Here's how the part is built. I have some questions about the finished solid (model axes, mm). Give positions to 0.01 mm unless a question says otherwise; leave off trailing zeros. Write each loop counter-clockwise with the first axis right and the second up, starting at its lowest first coordinate (ties: lowest second). Pieces come first, ordered by that corner, then holes. Notation, with made-up numbers: (10.5, -8.75) -> (19.5, -8.75) arc R15 cw to (19.5, 1.25) -> close; hole circle Ø11 at (44, -8.75). An arc over 180 degrees is marked (long way). Return JSON: item names as keys, results as strings.
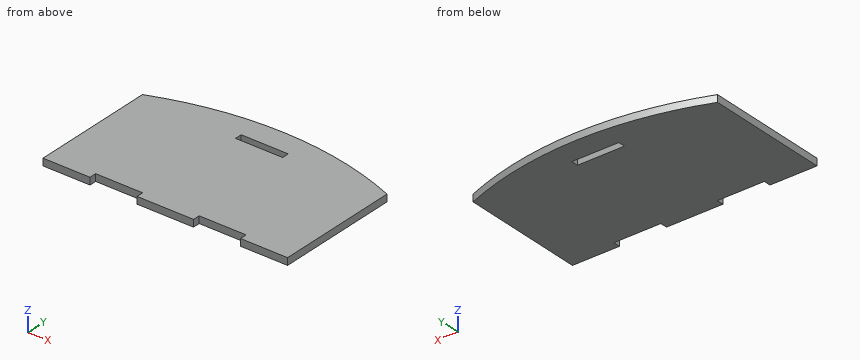
from build123d import *

# Parameters (mm, degrees)
SKETCH1_W           = 20
SKETCH1_H           = 3
BOSS_EXTRUDE1_DEPTH = 3


with BuildPart() as part:
    # Sketch1 → Boss-Extrude1 (new body)
    with BuildSketch(Plane.XY):
        with BuildLine():
            Line((-9.242159986, -25.403689193), (-9.242159986, -22.403689193))
            Line((-9.242159986, -22.403689193), (10.757840014, -22.403689193))
            Line((10.757840014, -22.403689193), (10.757840014, -25.403689193))
            Line((10.757840014, -25.403689193), (34.757840014, -25.403689193))
            Line((34.757840014, -25.403689193), (34.757840014, -22.403689193))
            Line((34.757840014, -22.403689193), (54.757840014, -22.403689193))
            Line((54.757840014, -22.403689193), (54.757840014, -25.403689193))
            Line((54.757840014, -25.403689193), (74.757840014, -25.403689193))
            Line((74.757840014, -25.403689193), (74.757840014, 27.596310807))
            ThreePointArc((74.757840014, 27.596310807), (22.757840014, 37.596310807), (-29.242159986, 27.596310807))
            Line((-29.242159986, 27.596310807), (-29.242159986, -25.403689193))
            Line((-29.242159986, -25.403689193), (-9.242159986, -25.403689193))
        make_face()
        with Locations((22.757840014, 26.096310807)):
            Rectangle(SKETCH1_W, SKETCH1_H, mode=Mode.SUBTRACT)
    extrude(amount=BOSS_EXTRUDE1_DEPTH)


solid = part.part
1. For pin 1 Ø0.9 at (x, z) = (19, 2) entering from +Y; pin 2 Ø2 at (x, y) = (35.5, -15) entering from -Z; pin 3 Ø1.5 at (x, z) = (-3, 2) entering from -Y, each with a flat end and sliding along its axis, tell me the tip position at first contact or that it passes through.
Taken from the geometry:
{"pin 1": "stops at y = 37.56", "pin 2": "stops at z = 0", "pin 3": "stops at y = -22.4"}
2. Suppose I cut it at C-C, the plane x = 68. List the corners of the cut face in (y, z) for me.
Taken from the geometry:
{"outline": "(-25.4, 0) -> (30.1, 0) -> (30.1, 3) -> (-25.4, 3) -> close"}
3. If I drill on line 1 (X direction, y = -23, z = 1.9); line 2 (X direction, y = 26, z = 1.25); line 3 (Y direction, x = 50.5, z = 1.75), over which ranges is the centre line in solid material (lowest first)? Write a range as [from, to].
Taken from the geometry:
{"line 1": "x = [-29.24, -9.24], [10.76, 34.76], [54.76, 74.76]", "line 2": "x = [-29.24, 12.76], [32.76, 74.76]", "line 3": "y = [-22.4, 34.82]"}
4. Suppose I cut it at D-D, the plane x = 51. List the corners of the cut face in (y, z) for me, and give its area (3 significant figures).
Taken from the geometry:
{"outline": "(-22.4, 0) -> (34.72, 0) -> (34.72, 3) -> (-22.4, 3) -> close", "area": "171 mm²"}
5. Suppose I cut it at B-B, the plane x = 23. List the corners of the cut face in (y, z) for me.
Taken from the geometry:
{"outline": "(-25.4, 0) -> (24.6, 0) -> (24.6, 3) -> (-25.4, 3) -> close; (27.6, 0) -> (37.6, 0) -> (37.6, 3) -> (27.6, 3) -> close"}
6. Suppose I cut it at A-A, the plane z = 1.2. List the corners of the cut face in (x, y) for me.
Taken from the geometry:
{"outline": "(-29.24, -25.4) -> (-9.24, -25.4) -> (-9.24, -22.4) -> (10.76, -22.4) -> (10.76, -25.4) -> (34.76, -25.4) -> (34.76, -22.4) -> (54.76, -22.4) -> (54.76, -25.4) -> (74.76, -25.4) -> (74.76, 27.6) arc R140.2 ccw to (-29.24, 27.6) -> close; hole (12.76, 24.6) -> (32.76, 24.6) -> (32.76, 27.6) -> (12.76, 27.6) -> close"}
